```python
from build123d import *

# Parameters (mm, degrees)
BOSS_EXTRUDE1_DEPTH     = 20
SKETCH3_R               = 3.3
CUT_EXTRUDE1_DEPTH      = 1
CUT_EXTRUDE1_DEPTH_BACK = 10
FILLET1_R               = 1
FILLET2_R               = 0.5
CHAMFER1_SIZE           = 0.25
SKETCH4_R               = 3.85
CUT_EXTRUDE2_DEPTH      = 1
SKETCH5_R               = 3.85
SKETCH5_R_2             = 3.75
CUT_EXTRUDE3_DEPTH      = 5
CHAMFER2_SIZE           = 0.25
CUT_EXTRUDE4_DEPTH      = 2.5
SKETCH7_R               = 2.5
BOSS_EXTRUDE2_DEPTH     = 1
SKETCH8_R               = 2.5
CUT_EXTRUDE5_DEPTH      = 1
SKETCH9_R               = 2.165063509
CUT_EXTRUDE6_DEPTH      = 1
CUT_EXTRUDE6_TAPER      = 45


with BuildPart() as part:
    # Sketch1 → Boss-Extrude1 (new body)
    with BuildSketch(Plane.XY):
        with BuildLine():
            Line((-30, 0), (30, 0))
            Line((30, 0), (30, 10))
            Line((30, 10), (15, 10))
            Line((15, 10), (15, 51))
            Line((15, 51), (0.5, 51))
            Line((0.5, 51), (0.5, 40.987492178))
            ThreePointArc((0.5, 40.987492178), (0, 21), (-0.5, 40.987492178))
            Line((-0.5, 40.987492178), (-0.5, 51))
            Line((-0.5, 51), (-15, 51))
            Line((-15, 51), (-15, 10))
            Line((-15, 10), (-30, 10))
            Line((-30, 10), (-30, 0))
        make_face()
    extrude(amount=BOSS_EXTRUDE1_DEPTH)

    # Sketch3 → Cut-Extrude1 (cut, two sides)
    with BuildSketch(Plane.XZ) as cut_extrude1_sk:
        with Locations((-22.5, 10)):
            Circle(SKETCH3_R)
        with Locations((22.5, 10)):
            Circle(SKETCH3_R)
    extrude(amount=CUT_EXTRUDE1_DEPTH, mode=Mode.SUBTRACT)
    extrude(cut_extrude1_sk.sketch, amount=-CUT_EXTRUDE1_DEPTH_BACK, mode=Mode.SUBTRACT)

    # Fillet1
    fillet1_edges = [part.edges().sort_by_distance(p)[0] for p in [
        (-30, 10, 10),
        (30, 10, 10),
    ]]
    fillet(fillet1_edges, radius=FILLET1_R)

    # Fillet2
    fillet2_edges = [part.edges().sort_by_distance(p)[0] for p in [
        (-15, 10, 10),
        (-15, 51, 10),
        (15, 51, 10),
        (15, 10, 10),
    ]]
    fillet(fillet2_edges, radius=FILLET2_R)

    # Chamfer1
    chamfer1_edges = [part.edges().sort_by_distance(p)[0] for p in [
        (0, 21, 0),
        (0, 21, 20),
        (19.2, 10, 10),
        (19.2, 0, 10),
        (-25.8, 10, 10),
        (-25.8, 0, 10),
    ]]
    chamfer(chamfer1_edges, length=CHAMFER1_SIZE)

    # Sketch4 → Cut-Extrude2 (cut)
    with BuildSketch(Plane.ZY.offset(15)):
        with Locations((10, 46)):
            Circle(SKETCH4_R)
    extrude(amount=-CUT_EXTRUDE2_DEPTH, mode=Mode.SUBTRACT)

    # Sketch5 → Cut-Extrude3 (cut)
    with BuildSketch(Plane.ZY.offset(14)):
        with Locations((10, 46)):
            Circle(SKETCH5_R)
        with Locations((10, 46)):
            Circle(SKETCH5_R_2, mode=Mode.SUBTRACT)
    extrude(amount=-CUT_EXTRUDE3_DEPTH, mode=Mode.SUBTRACT)

    # Chamfer2
    chamfer2_edges = [part.edges().sort_by_distance(p)[0] for p in [
        (-14, 46, 6.25),
    ]]
    chamfer(chamfer2_edges, length=CHAMFER2_SIZE)

    # Sketch6 → Cut-Extrude4 (cut)
    with BuildSketch(Plane.ZY.offset(14)):
        Polygon((9.85568838, 43.839751367), (11.798674385, 44.794898154), (11.942986005, 46.955146787), (10.14431162, 48.160248633), (8.201325615, 47.205101846), (8.057013995, 45.044853213), align=None)
    extrude(amount=-CUT_EXTRUDE4_DEPTH, mode=Mode.SUBTRACT)

    # Sketch7 → Boss-Extrude2 (add)
    with BuildSketch(Plane(origin=(-0.5, 0, 0), x_dir=(0, 0, -1), z_dir=(1, 0, 0))):
        with Locations((-10, 46)):
            Circle(SKETCH7_R)
    extrude(amount=BOSS_EXTRUDE2_DEPTH)

    # Sketch8 → Cut-Extrude5 (cut)
    with BuildSketch(Plane(origin=(15, 0, 0), x_dir=(0, 0, -1), z_dir=(1, 0, 0))):
        with Locations((-10, 46)):
            Circle(SKETCH8_R)
    extrude(amount=-CUT_EXTRUDE5_DEPTH, mode=Mode.SUBTRACT)

    # Sketch9 → Cut-Extrude6 (cut)
    with BuildSketch(Plane.ZY.offset(14)):
        with Locations((10, 46)):
            Circle(SKETCH9_R)
    extrude(amount=-CUT_EXTRUDE6_DEPTH, taper=CUT_EXTRUDE6_TAPER, mode=Mode.SUBTRACT)


solid = part.part
```
For this review, take the finished solid that the model builds, in its own axes (mm). A direction names the side the tool comes from. Give positions to 0.01 mm unless a question says otherwise; leave off trailing zeros. Loops run counter-clockwise (first coordinate to the right, second up) from the corner with the lowest first, then second, coordinate; pieces in that order, holes last. Notation, with made-up numbers: M -7,35.25 L -1,35.25 A22 ccw -1,50.25 Z; hole C 89.5,59.25 d8. An arc over 180 degrees is marked long. One line per item, written item: value. Start each with the question number.
Q1. For L1, parallel to Y at x = 14.2, z = 10; L2, parallel to X at y = 48, z = 17.5; L3, parallel to Z at x = -22.5, y = 2.5, list the stretches that pass through material, from the lowest coordinate up.
Q2. Add section C-C (z = 15). Give the boundary of the cut face in (x, y), and give its area (3 significant figures).
Q3. Clearance check with flat-ended pins moving along their axes: pin 1 Ø6 at (y, z) = (21, 13) entering from -X; pin 2 Ø4 at (x, z) = (-25, 5.5) entering from +Y; pin 3 Ø6.5 at (y, z) = (46, 10) entering from -X. State where each tip first meets the part, or that it passes through.
Q4. Draft analysis for pull direction X (two halves, no side actions). For faces 4 (the face through (-12.768, 47.549, 11.056)), 5 (the face through (-14, 48, 12)), 6 (the face through (30, 4, 10)), 7 (the face through (-0.5, 44.8, 7.6)), state which applies: released by +X, released by -X, zero draft, split by the parting line, or undercut.
Q5. Add section D-D (x = -17). Give the boundary of the cut face in (y, z), and give its area (3 significant figures).
Q6. Add section B-B (x = 22.5). Give the boundary of the cut face in (y, z), and give its area (3 significant figures).
Q7. Machinability: for faces 1 (the face through (-12.768, 44.451, 8.944)), 2 (the face through (19, 10, 8)), 3 (the face through (-15, 31, 10)), which of the approach directions +Z, -Z, +X, -X, +Y, -Y give a long, thin tool a straight path to every point of the face, cutting with its end or side? Answer none if there is none.
Q8. Add section A-A (y = 31). Give the boundary of the cut face in (x, z).
Reply:
1. L1: 0 to 43.5, 48.5 to 51
1. L2: -15 to -0.5, 0.5 to 15
1. L3: 0 to 6.7, 13.3 to 20
2. outline: M -30,0 L 30,0 L 30,9 A1 ccw 29,10 L 15.5,10 A0.5 cw 15,10.5 L 15,50.5 A0.5 ccw 14.5,51 L 0.5,51 L 0.5,40.99 A10 cw long -0.5,40.99 L -0.5,51 L -14.5,51 A0.5 ccw -15,50.5 L -15,10.5 A0.5 cw -15.5,10 L -29,10 A1 ccw -30,9 Z
2. area: 1,510 mm²
3. pin 1: x = -15
3. pin 2: y = 10
3. pin 3: x = -14
4. face 4: zero draft
4. face 5: released by -X
4. face 6: released by +X
4. face 7: undercut
5. outline: M 0,0 L 10,0 L 10,20 L 0,20 Z
5. area: 200 mm²
6. outline: M 0,0 L 10,0 L 10,6.45 L 9.75,6.7 L 0.25,6.7 L 0,6.45 Z; M 0,13.55 L 0.25,13.3 L 9.75,13.3 L 10,13.55 L 10,20 L 0,20 Z
6. area: 134 mm²
7. face 1: -X
7. face 2: +Z, -Z, +X, +Y
7. face 3: +Z, -Z, -X, +Y
8. outline: M -15,0 L -10.25,0 L -10,0.25 L -10,19.75 L -10.25,20 L -15,20 Z; M 10,0.25 L 10.25,0 L 15,0 L 15,20 L 10.25,20 L 10,19.75 Z
